from build123d import *

# Parameters (mm, degrees)
F2_DEPTH = 1
F3_SIZE  = 5
F4_SIZE  = 0.5


with BuildPart() as f2:
    # F1 (on face) → F2 (new body)
    with BuildSketch(Plane.XY):
        Polygon((-47, 12.5), (-47, -3.5), (-38, -3.5), (-38, -12.5), (-32, -12.5), (-32, -3.5), (-28, -3.5), (-28, -12.5), (-22, -12.5), (-22, -3.5), (-18, -3.5), (-18, -12.5), (-12, -12.5), (-12, -3.5), (-8, -3.5), (-8, -12.5), (-2, -12.5), (-2, -3.5), (2, -3.5), (2, -12.5), (8, -12.5), (8, -3.5), (12, -3.5), (12, -12.5), (18, -12.5), (18, -3.5), (22, -3.5), (22, -12.5), (28, -12.5), (28, -3.5), (32, -3.5), (32, -12.5), (38, -12.5), (38, -3.5), (47, -3.5), (47, 12.5), align=None)
    extrude(amount=F2_DEPTH)

    # F3
    f3_edges = [f2.edges().sort_by_distance(p)[0] for p in [
        (47, 12.5, 0.5),
        (-47, 12.5, 0.5),
    ]]
    chamfer(f3_edges, length=F3_SIZE)

    # F4
    f4_edges = [f2.edges().sort_by_distance(p)[0] for p in [
        (-47, 2, 0),
        (-44.5, 10, 0),
        (-42.5, -3.5, 0),
        (0, 12.5, 0),
        (-38, -8, 0),
        (44.5, 10, 0),
        (-35, -12.5, 0),
        (47, 2, 0),
        (-32, -8, 0),
        (42.5, -3.5, 0),
        (-30, -3.5, 0),
        (38, -8, 0),
        (-28, -8, 0),
        (35, -12.5, 0),
        (-25, -12.5, 0),
        (32, -8, 0),
        (-22, -8, 0),
        (30, -3.5, 0),
        (-20, -3.5, 0),
        (28, -8, 0),
        (-18, -8, 0),
        (25, -12.5, 0),
        (-15, -12.5, 0),
        (22, -8, 0),
        (-12, -8, 0),
        (20, -3.5, 0),
        (-10, -3.5, 0),
        (18, -8, 0),
        (-8, -8, 0),
        (15, -12.5, 0),
        (-5, -12.5, 0),
        (12, -8, 0),
        (-2, -8, 0),
        (10, -3.5, 0),
        (0, -3.5, 0),
        (8, -8, 0),
        (2, -8, 0),
        (5, -12.5, 0),
    ]]
    chamfer(f4_edges, length=F4_SIZE)


solid = f2.part
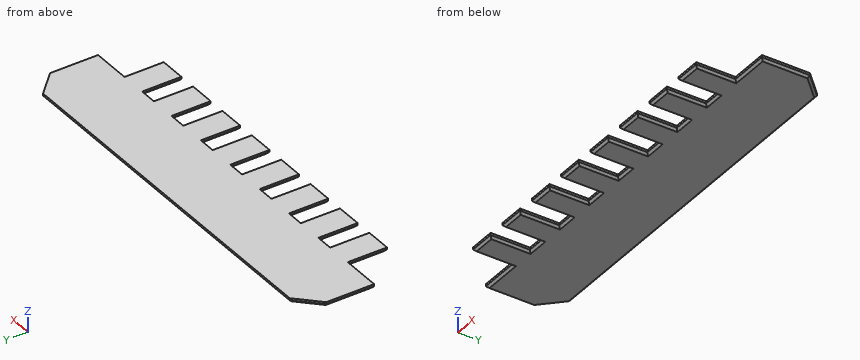
Build history of the part. All positions in model axes, mm. Give positions to 0.01 mm unless a question says otherwise; leave off trailing zeros. Write each loop counter-clockwise with the first axis right and the second up, starting at its lowest first coordinate (ties: lowest second). Pieces come first, ordered by that corner, then holes. Notation, with made-up numbers: (-20.75, -36.75) - (-0.75, -36.75) arc R18 cw to (-0.75, -22.75) - close; hole circle Ø2 at (-20, 34). An arc over 180 degrees is marked (long way). Use one line per item in the form item = value. Start each with the question number.
1. Band-saw the part on A-A on y = -7. Count the separate pieces of the cut face and the enclosed holes in it, plus the area to 3 significant figures.
2. Probe line 1 (Y direction, x = -0.5, z = 0.7); line 2 (X direction, y = 0.5, z = 0.3); line 3 (Y direction, x = -33, z = 0.25). List the from-to ranges inside material, lowest first. Write a range as [from, to].
3. Band-saw the part on B-B on x = 39.5. Write the cut outline in (y, z), plus the area to 4 significant figures.
4. Drop flat-ended pins along their axis: pin 1 Ø0.6 at (y, z) = (-9.5, 0.5) entering from +X; pin 2 Ø0.6 at (x, z) = (0, 1) entering from -Y. Give the stop position or say it passes through.
Conclusion:
q1.separate_pieces = 8
q1.enclosed_holes = 0
q1.area = 46.0 mm²
q2.line_1 = [-3.5, 12.5]
q2.line_2 = [-46.8, 46.8]
q2.line_3 = [-12.25, 12.25]
q3.outline = (-3.5, 0.5) - (-3, 0) - (12, 0) - (12.5, 0.5) - (12.5, 1) - (-3.5, 1) - close
q3.area = 15.75 mm²
q4.pin_1 = 38
q4.pin_2 = -3.5
